```python
from build123d import *

# Parameters (mm, degrees)
PAD021_DEPTH      = 5
BOX002_W          = 5.4
BOX002_H          = 5.4
BOX002_DEPTH      = 4
CYLINDER063_R     = 2.25
CYLINDER063_DEPTH = 9
SKETCH034_R       = 4.5
POCKET004_DEPTH   = 2.5


with BuildPart() as part:
    # Sketch031 → Pad021 (new body)
    with BuildSketch(Plane.XZ):
        with BuildLine():
            ThreePointArc((-18, 8), (-26, 0), (-18, -8))
            Line((-18, -8), (-8.944272, -8))
            ThreePointArc((-8.944272, 8), (-12, 0), (-8.944272, -8))
            Line((-18, 8), (-8.944272, 8))
        make_face()
    extrude(amount=PAD021_DEPTH)

    # Box002 → Box002 (join)
    with BuildSketch(Plane(origin=(-20.7, 4, -2.7), x_dir=(1, 0, 0), z_dir=(0, -1, 0))):
        with Locations((2.7, 2.7)):
            Rectangle(BOX002_W, BOX002_H)
    extrude(amount=BOX002_DEPTH)

    # Cylinder063 → Cylinder063 (cut)
    with BuildSketch(Plane(origin=(-18, 4, 0), x_dir=(1, 0, 0), z_dir=(0, -1, 0))):
        Circle(CYLINDER063_R)
    extrude(amount=CYLINDER063_DEPTH, mode=Mode.SUBTRACT)

    # Sketch034 (on Face5 of Cylinder063) → Pocket004 (cut)
    with BuildSketch(Plane(origin=(-18, -5, 0), x_dir=(1, 0, 0), z_dir=(0, -1, 0))):
        Circle(SKETCH034_R)
    extrude(amount=-POCKET004_DEPTH, mode=Mode.SUBTRACT)


with BuildPart() as part_1:
    # Body033 placement: moved
    add(part.part.moved(Location((0, -5, 0))))


solid = part_1.part
```
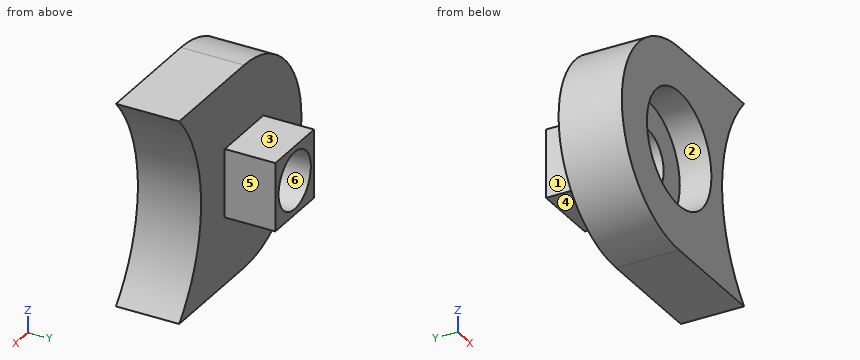
Geometry: final body of the model. Coordinates: model frame, mm. Face numbers are marked on the shaded views. A direction names the side the tool comes from. Coordinates: 2 decimals unless noted, no trailing zeros. Order: outer loops, then holes, each group sorted by start corner. A loop starts at its lowest first (then second) coordinate and runs counter-clockwise, first axis right, second up. Notation, with made-up numbers: (0, 69.25) - (9, 69.25) arc R5 cw to (9, 78.25) - close; hole circle Ø1 at (58, -2). An arc over 180 degrees is marked (long way). Write each question's results on one line, items separated by ' | '.
1) Section D-D, the plane z = 4.25. Return loops of the section in (x, y), plus the area to 3 significant figures.
Results list:
outline: (-24.78, -10) - (-19.48, -10) - (-19.48, -7.5) - (-16.52, -7.5) - (-16.52, -10) - (-11.22, -10) - (-11.22, -5) - (-24.78, -5) - close | area: 60.4 mm^2
2) Pull-direction query (Z, two-part tool) for the marked faces 4, 5 and 6; classes: pulls with the +Z half, pulls with the -Z half, needs draft (parallel to the pull), parting line crosses it, or undercut.
Results list:
face 4: pulls with the -Z half | face 5: needs draft | face 6: undercut
3) Section A-A, the plane y = -9.25. Return loops of the section in (x, z), plus the area to 3 significant figures.
Results list:
outline: (-18, -8) - (-8.94, -8) arc R12 cw to (-8.94, 8) - (-18, 8) arc R8 ccw to start; hole circle Ø9 at (-18, 0) | area: 148 mm^2
4) Pin query (flat end, axial travel): pin 1 (1.5 mm diameter, centred on x = -20.5, y = -5, fed in from +Z); pin 2 (5.5 mm diameter, centred on x = -18, z = 0, fed in from -Y); pin 3 (4.5 mm diameter, centred on y = -2.5, z = -1, fed in from -X); pin 4 (3.5 mm diameter, centred on x = -18, z = 0, fed in from +Y). Return the tip coordinate at first contact, or that it passes through.
Results list:
pin 1: z = 7.81 | pin 2: y = -7.5 | pin 3: x = -20.7 | pin 4: through
5) Section C-C, the plane x = -20. Return loops of the section in (y, z).
Results list:
outline: (-10, -7.75) - (-5, -7.75) - (-5, -2.7) - (-1, -2.7) - (-1, -1.03) - (-7.5, -1.03) - (-7.5, -4.03) - (-10, -4.03) - close; (-10, 4.03) - (-7.5, 4.03) - (-7.5, 1.03) - (-1, 1.03) - (-1, 2.7) - (-5, 2.7) - (-5, 7.75) - (-10, 7.75) - close
6) Set-up query: the marked faces 1, 2 and 3. Return all of +Z, -Z, +X, -X, +Y, -Y with unobstructed straight access to the full face (end or side cutting, diameter ignored); none if empty.
Results list:
face 1: +Z, -Z, -X, +Y | face 2: -Y | face 3: +Z, +X, -X, +Y
7) Section B-B, the plane z = 0. Return loops of the section in (x, y), plus the area to 4 significant figures.
Results list:
outline: (-26, -10) - (-22.5, -10) - (-22.5, -7.5) - (-20.25, -7.5) - (-20.25, -1) - (-20.7, -1) - (-20.7, -5) - (-26, -5) - close; (-15.75, -7.5) - (-13.5, -7.5) - (-13.5, -10) - (-12, -10) - (-12, -5) - (-15.3, -5) - (-15.3, -1) - (-15.75, -1) - close | area: 39.85 mm^2
8) Line query: line 1 (Z direction, x = -18, y = -2.5); line 2 (Z direction, x = -18, y = -5.5); line 3 (Y direction, x = -17.5, z = 5). Output: solid intervals per line, ascending. Write a range as from..to.
Results list:
line 1: -2.7..-2.25, 2.25..2.7 | line 2: -8..-2.25, 2.25..8 | line 3: -10..-5
